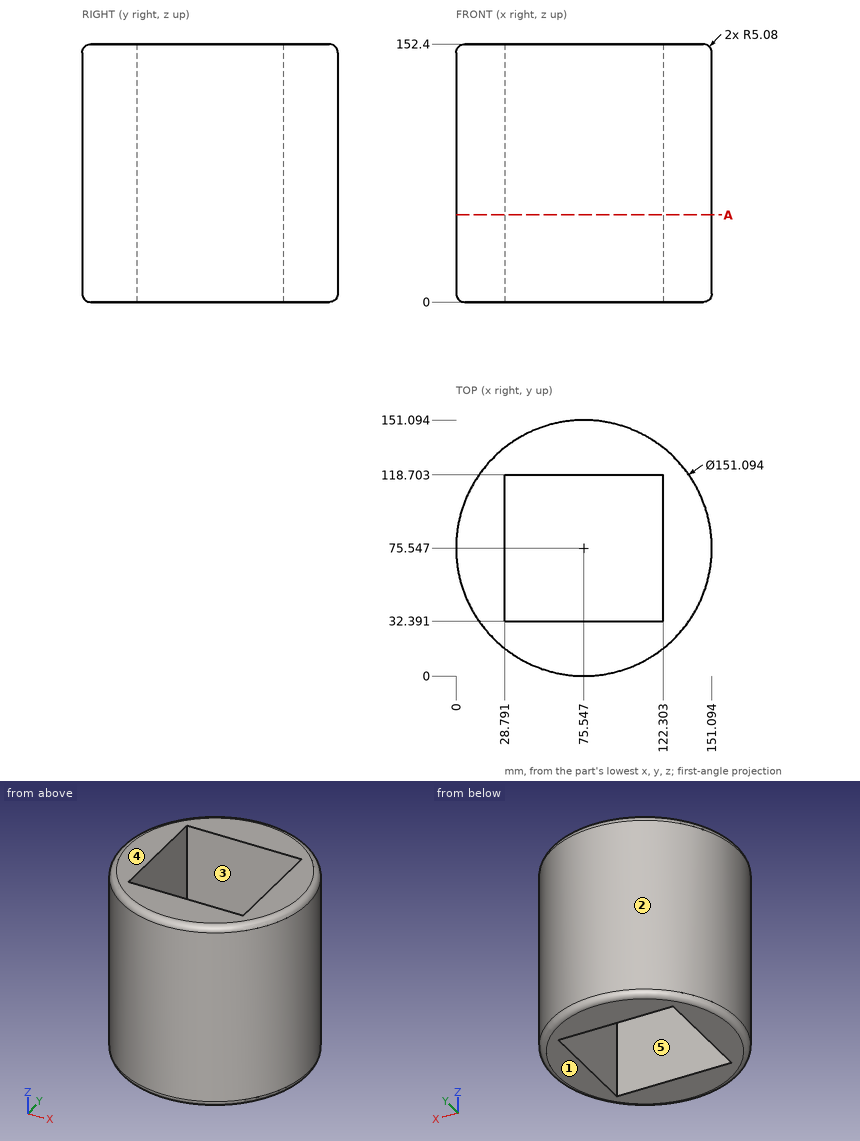
For this review, use the dimensioned drawing (mm, ordinates from the lowest corner) and the shaded views. A direction names the side the tool comes from. Give positions to 0.01 mm unless a question says otherwise; leave off trailing zeros. Loops run counter-clockwise (first coordinate to the right, second up) from the corner with the lowest first, then second, coordinate; pieces in that order, holes last. Notation, with made-up numbers: (-20, 3) -> (12, 3) arc R36 cw to (12, 38) -> close; hole circle Ø2 at (37, 75). An arc over 180 degrees is marked (long way). Use CSV: the item, a comma, the result in double quotes.
1. For P1, Ø2, axis at x = 53.5, z = 73.5, coming from the +Y side; P2, Ø8, axis at y = 27, z = 58, coming from the -X side; P3, Ø8, axis at y = 71, z = 102, coming from the +X side, all flat-tipped, find the tip position at first contact; note any pin that passes through.
Result:
P1,"stops at y = 148.1"
P2,"stops at x = 14.53"
P3,"stops at x = 151.09"
2. Machinability: for the marked faces 4 and 5, which of the approach directions +Z, -Z, +X, -X, +Y, -Y give a long, thin tool a straight path to every point of the face, cutting with its end or side? Answer none if there is none.
Result:
face 4,"+Z, +X, -X, +Y, -Y"
face 5,"+Z, -Z"
3. To check wall thickness, follow probe 1 along X at (y, z) = (95.5, 28); probe 2 along X at (y, z) = (45, 69.5); probe 3 along Y at (x, z) = (109, 136) (1 decimal). State the ranges of each line that lie inside material, in increasing order. Write a range as from..to.
Result:
probe 1,"x = 2.68..28.79, 122.3..148.41"
probe 2,"x = 6.45..28.79, 122.3..144.64"
probe 3,"y = 7.8..32.4, 118.7..143.3"
4. The part is to be moulded in two halves that separate along Y. For the marked faces 1, 2 and 3, say which applies: +Y half, -Y half, draft (parallel to the pull), parting line (faces both ways), or undercut.
Result:
face 1,"draft"
face 2,"parting line"
face 3,"undercut"
5. Consider section A-A, the plane z = 51.5. Write out the cut boundary in (x, y) (1 decimal).
Result:
outline,"circle Ø151.1 at (75.5, 75.5); hole (28.8, 32.4) -> (122.3, 32.4) -> (122.3, 118.7) -> (28.8, 118.7) -> close"
